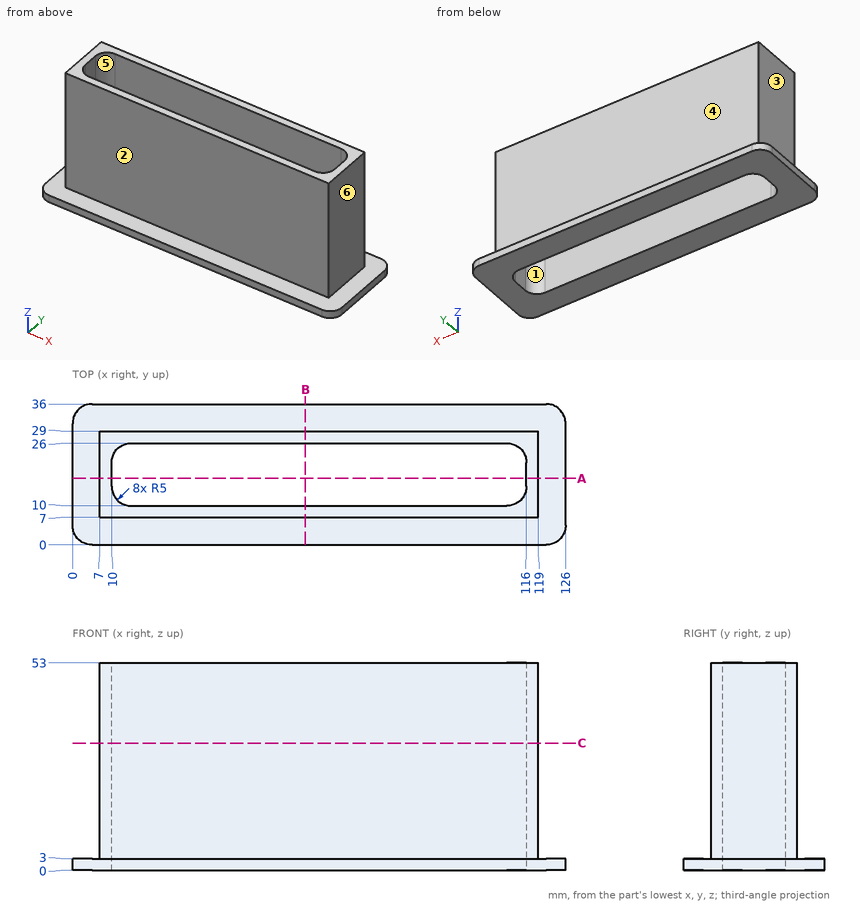
Could you check a few things on this drawing? It's one solid part, dimensions in mm from its lowest x, y, z. A direction names the side the tool comes from. Coordinates: 2 decimals unless noted, no trailing zeros. Order: outer loops, then holes, each group sorted by start corner. A loop starts at its lowest first (then second) coordinate and runs counter-clockwise, first axis right, second up.
1. If we section it at A-A (y = 17): Please give me the cut outline in (x, z).
2. If we section it at B-B (x = 59.5): Please give me the cut outline in (y, z).
3. I'm going to push flat-ended pins straight in: pin 1 (1.5 mm diameter, centred on y = 28, z = 12, fed in from -X); pin 2 (16 mm diameter, centred on x = 79, z = 32.5, fed in from -Y); pin 3 (5 mm diameter, centred on y = 17, z = 36.5, fed in from +X). Where does each tip first touch, or does it pass through?
4. For the marked faces 1, 2 and 3, which set-ups out of +Z, -Z, +X, -X, +Y, -Y let a thin tool reach every point of the face, with its end or its side?
5. I need wall thicknesses on line 1 (Y direction, x = 20, z = 14.5); line 2 (X direction, y = 18, z = 25); line 3 (Z direction, x = 113, y = 32.5). Which ranges of each line are inside material? Lowest first, please.
6. Thinking about a two-plate mould opening in X: for the marked faces 4, 5 and 6, which applies, +X half, -X half, draft (parallel to the pull), parting line (faces both ways), or undercut?
7. If we section it at C-C (z = 32.5): Please give me the cut outline in (x, y).
Entries:
1. outline: (0, 0) - (10, 0) - (10, 53) - (7, 53) - (7, 3) - (0, 3) - close; (116, 0) - (126, 0) - (126, 3) - (119, 3) - (119, 53) - (116, 53) - close
2. outline: (0, 0) - (10, 0) - (10, 53) - (7, 53) - (7, 3) - (0, 3) - close; (26, 0) - (36, 0) - (36, 3) - (29, 3) - (29, 53) - (26, 53) - close
3. pin 1: stops at x = 7
3. pin 2: stops at y = 7
3. pin 3: stops at x = 119
4. face 1: +Z, -Z
4. face 2: +Z, +X, -X, -Y
4. face 3: +Z, -X, +Y, -Y
5. line 1: y = 7 to 10, 26 to 29
5. line 2: x = 7 to 10, 116 to 119
5. line 3: z = 0 to 3
6. face 4: draft
6. face 5: undercut
6. face 6: +X half
7. outline: (7, 7) - (119, 7) - (119, 29) - (7, 29) - close; hole (10, 15) arc R5 ccw to (15, 10) - (111, 10) arc R5 ccw to (116, 15) - (116, 21) arc R5 ccw to (111, 26) - (15, 26) arc R5 ccw to (10, 21) - close
